Part print with two shaded views. Sizes in mm from the minimum x, y, z corner. A direction names the side the tool comes from. Round coordinates to 2 decimals unless told otherwise and drop trailing zeros. Order: outer loops, then holes, each group sorted by start corner. A loop starts at its lowest first (then second) coordinate and runs counter-clockwise, first axis right, second up. Notation, with made-up numbers: M -37.75,67 L 17.25,67 A25 ccw 17.25,92 Z; hole C 30,60.25 d1. An arc over 180 degrees is marked long. Return JSON: item names as keys, results as strings. Group by question number.
Item 1: Which spindle directions (+Z, -Z, +X, -X, +Y, -Y) get a long thin tool onto all of the face, cutting with end or side? Do the marked faces 4 and 5. Say none if no direction does.
Item 2: Slice it at A-A on y = 37.5. Write the cut outline in (x, z), then the cut area to 3 significant figures.
Item 3: Slice it at D-D on y = 16. Write the cut outline in (x, z) (1 decimal), then the cut area to 3 significant figures.
Item 4: Slice it at B-B on x = 37.5. Write the cut outline in (y, z), then the cut area to 3 significant figures.
Item 5: Probe line 1 along Y through (x, z) = (37.5, 12.25); line 2 along Z through (x, y) = (56, 17); line 3 along Y through (x, z) = (37.5, 2.4). List the from-to ranges inside material, lowest first.
Item 6: Slice it at C-C on x = 21. Write the cut outline in (y, z) (1 decimal), then the cut area to 3 significant figures.
Item 7: Pin check, flat tips, straight feed: pin 1 Ø2 at (x, z) = (28.5, 17) entering from -Y; pin 2 Ø6.5 at (x, y) = (71.8, 37.5) entering from -Z; pin 3 Ø1.5 at (x, z) = (33, 16.5) entering from -Y; pin 4 Ø1.5 at (y, z) = (20, 8.5) entering from +X. Stop position of each tip, or through.
Item 8: Pull direction Y, two halves, no side cores. Call the marked faces 1, 2 and 3: pulls with the +Y half, pulls with the -Y half, needs draft (parallel to the pull), parting line crosses it, or undercut.
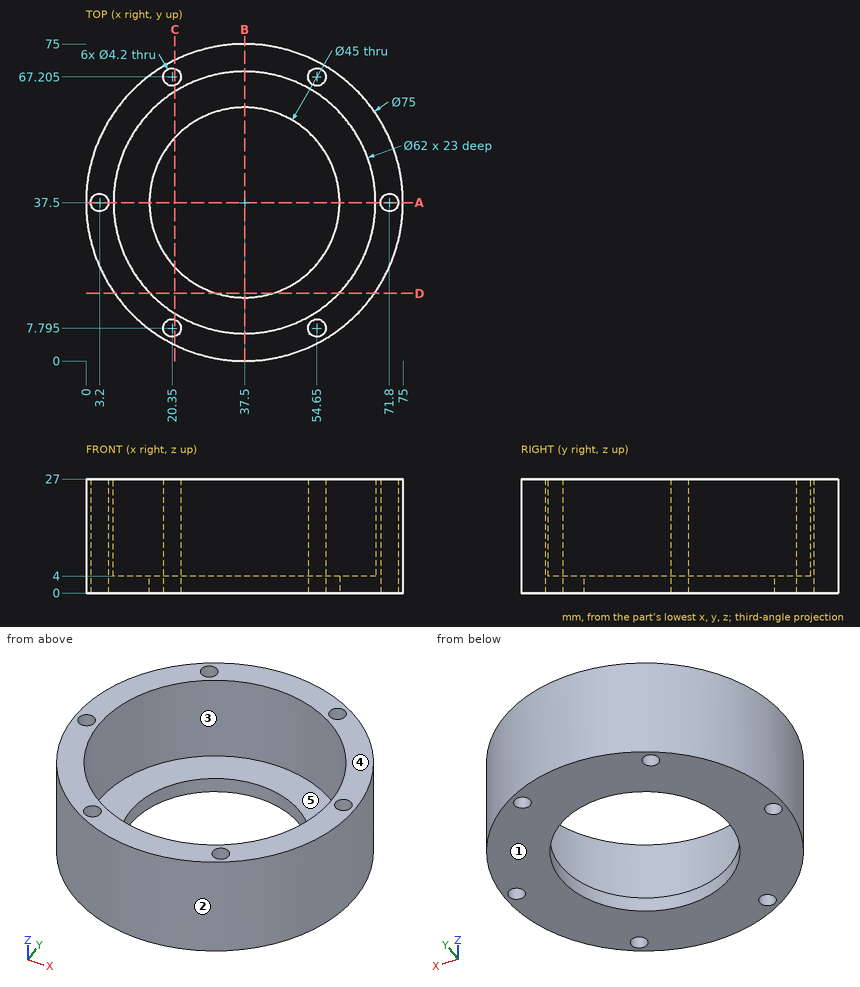
Output values:
{
 "1": {"face 4": "+Z, +X, -X, +Y, -Y", "face 5": "+Z"},
 "2": {"outline": "M 0,0 L 1.1,0 L 1.1,27 L 0,27 Z; M 5.3,0 L 15,0 L 15,4 L 6.5,4 L 6.5,27 L 5.3,27 Z; M 60,0 L 69.7,0 L 69.7,27 L 68.5,27 L 68.5,4 L 60,4 Z; M 73.9,0 L 75,0 L 75,27 L 73.9,27 Z", "area": "192 mm²"},
 "3": {"outline": "M 6.8,0 L 30.9,0 L 30.9,4 L 15.2,4 L 15.2,27 L 6.8,27 Z; M 44.1,0 L 68.2,0 L 68.2,27 L 59.8,27 L 59.8,4 L 44.1,4 Z", "area": "579 mm²"},
 "4": {"outline": "M 0,0 L 15,0 L 15,4 L 6.5,4 L 6.5,27 L 0,27 Z; M 60,0 L 75,0 L 75,27 L 68.5,27 L 68.5,4 L 60,4 Z", "area": "419 mm²"},
 "5": {"line 1": "0 to 6.5, 68.5 to 75", "line 2": "0 to 4", "line 3": "0 to 15, 60 to 75"},
 "6": {"outline": "M 3.8,0 L 5.8,0 L 5.8,27 L 3.8,27 Z; M 9.8,0 L 22.2,0 L 22.2,4 L 11.3,4 L 11.3,27 L 9.8,27 Z; M 52.8,0 L 65.2,0 L 65.2,27 L 63.7,27 L 63.7,4 L 52.8,4 Z; M 69.2,0 L 71.2,0 L 71.2,27 L 69.2,27 Z", "area": "273 mm²"},
 "7": {"pin 1": "y = 0.86", "pin 2": "z = 0", "pin 3": "y = 0.19", "pin 4": "x = 71.05"},
 "8": {"face 1": "needs draft", "face 2": "parting line crosses it", "face 3": "undercut"}
}
